from build123d import *
from build123d import SkipClean  # not in build123d's __all__

# Parameters (mm, degrees)
F0_R         = 8.117177454
F1_DEPTH     = 25
F2_SIZE      = 3
F3_DEPTH     = 25
F4_SIZE      = 5
F5_T4_DEPTH  = 109.868464735
F5_S5_R      = 25
F5_T6_DEPTH  = 57
F5_T8_ANGLE  = 167.4336377222
F5_T12_DEPTH = 109.868464735
F5_S13_R     = 25
F5_T14_DEPTH = 57


# Not quite as in the source:
# - a fillet or chamfer that OpenCascade refuses, or shapes differently, is made with other operations: its cross-section is extruded or revolved along the edge and cut away or added


with BuildPart() as f1:
    # F0 (on Front) → F1 (new body)
    with BuildSketch(Plane.XZ):
        with BuildLine():
            ThreePointArc((5.4392563458, -24.4011165811), (19.5061709293, -15.6367930113), (25, 0))
            ThreePointArc((25, 0), (19.5061709293, 15.6367930113), (5.4392563458, 24.4011165811))
            ThreePointArc((5.4392563458, 24.4011165811), (-25, 0), (5.4392563458, -24.4011165811))
        make_face()
        Circle(F0_R, mode=Mode.SUBTRACT)
        with BuildLine():
            ThreePointArc((5.4392563458, 24.4011165811), (19.5061709293, 15.6367930113), (25, 0))
            ThreePointArc((25, 0), (19.5061709293, -15.6367930113), (5.4392563458, -24.4011165811))
            Line((5.4392563458, -24.4011165811), (91.6416380189, -14.909896868))
            ThreePointArc((91.6416380189, -14.909896868), (75, 0), (91.6416380189, 14.909896868))
            Line((91.6416380189, 14.909896868), (5.4392563458, 24.4011165811))
        make_face()
        with BuildLine():
            ThreePointArc((105, 0), (101.1719418698, 10.0093813424), (91.6416380189, 14.909896868))
            ThreePointArc((91.6416380189, 14.909896868), (75, 0), (91.6416380189, -14.909896868))
            ThreePointArc((91.6416380189, -14.909896868), (101.1719418698, -10.0093813424), (105, 0))
        make_face()
        with Locations((90, 0)):
            Circle(F0_R, mode=Mode.SUBTRACT)
    extrude(amount=F1_DEPTH)

    # F2
    f2_edges = [f1.edges().sort_by_distance(p)[0] for p in [
        (-25, -25, 0),
        (48.540447, -25, -19.655507),
        (105, -25, 0),
        (48.540447, -25, 19.655507),
        (-8.117177, -25, 0),
        (81.882823, -25, 0),
    ]]
    chamfer(f2_edges, length=F2_SIZE)

    # F0 (on Front) → F3 (join)
    with BuildSketch(Plane.XZ):
        with BuildLine():
            ThreePointArc((5.4392563458, -24.4011165811), (19.5061709293, -15.6367930113), (25, 0))
            ThreePointArc((25, 0), (19.5061709293, 15.6367930113), (5.4392563458, 24.4011165811))
            ThreePointArc((5.4392563458, 24.4011165811), (-25, 0), (5.4392563458, -24.4011165811))
        make_face()
        Circle(F0_R, mode=Mode.SUBTRACT)
    with SkipClean():  # cleaning this boolean's faces spoils the solid; the shape is the same uncleaned
        extrude(amount=-F3_DEPTH)

    # F4
    f4_edges = [f1.edges().sort_by_distance(p)[0] for p in [
        (-5.439256, 25, 24.401117),
        (-8.117177, 25, 0),
    ]]
    chamfer(f4_edges, length=F4_SIZE)

    # F5: chamfer of 3 on 1 edges, made by hand


with BuildPart() as f5_tool2:
    # F5_s3 → F5_t4 (new body)
    with BuildSketch(Plane(origin=(88.922009846, 0, -9.7906614225), x_dir=(0, 1, 0), z_dir=(-0.9939931245, 0, 0.1094425346))):
        Polygon((0, -21.8498281134), (-3, -24.8498281134), (0, -24.8498281134), align=None)
    extrude(amount=F5_T4_DEPTH)

    # F5_s5 → F5_t6 (cut, symmetric)
    with BuildSketch(Plane.XZ.offset(1.5)):
        Circle(F5_S5_R)
    extrude(amount=F5_T6_DEPTH, both=True, mode=Mode.SUBTRACT)


with BuildPart() as f1_1:
    add(f1.part, clean=False)

    # F5_t1: cut F5_tool2
    add(f5_tool2.part, mode=Mode.SUBTRACT)

    # F5_s7 → F5_t8 (revolve, cut)
    with BuildSketch(Plane(origin=(88.922009846, 0, 9.7906614225), x_dir=(0, 1, 0), z_dir=(-0.9939931245, 0, -0.1094425346))):
        Polygon((0, 21.8498281134), (-3, 24.8498281134), (0, 24.8498281134), align=None)
    revolve(axis=Axis((90, 0, 0), (0, -1, 0)), revolution_arc=F5_T8_ANGLE, mode=Mode.SUBTRACT)


with BuildPart() as f5_tool10:
    # F5_s11 → F5_t12 (new body)
    with BuildSketch(Plane(origin=(-20.2864887038, 0, -2.2336218299), x_dir=(0, 1, 0), z_dir=(0.9939931245, 0, 0.1094425346))):
        Polygon((0, -21.8498281134), (-3, -24.8498281134), (0, -24.8498281134), align=None)
    extrude(amount=F5_T12_DEPTH)

    # F5_s13 → F5_t14 (cut, symmetric)
    with BuildSketch(Plane.XZ.offset(1.5)):
        Circle(F5_S13_R)
    extrude(amount=F5_T14_DEPTH, both=True, mode=Mode.SUBTRACT)


with BuildPart() as f1_2:
    add(f1_1.part, clean=False)

    # F5_t9: cut F5_tool10
    add(f5_tool10.part, mode=Mode.SUBTRACT)


solid = f1_2.part
CAD build for the part. Positions are in the model's coordinates, mm. Give positions to 0.01 mm unless a question says otherwise; leave off trailing zeros. Write each loop counter-clockwise with the first axis right and the second up, starting at its lowest first coordinate (ties: lowest second). Pieces come first, ordered by that corner, then holes. Notation, with made-up numbers: M 74.25,-13 L 116.25,-13 A27 ccw 116.25,23 Z; hole C 61,-14 d10. An arc over 180 degrees is marked long. Put each result on its own line as item: value. Start each with the question number.
(1) Band-saw the part on C-C, the plane x = 45.5. Write the cut outline in (y, z).
(2) Flat gauge pins, fed straight in: pin 1 Ø6 at (x, y) = (46, -3.5) entering from -Z; pin 2 Ø3 at (x, y) = (57.5, -16) entering from +Z; pin 3 Ø10 at (y, z) = (-15.5, -13.5) entering from -X. Where does each tip first touch, or does it go through?
(3) Band-saw the part on B-B, the plane y = -17.5. Write the cut outline in (x, z).
(4) Mould opens along Z. For faces 1 (the face through (81.89, -10.85, 0.36)), 2 (the face through (105, -12, 0)), 3 (the face through (49.14, -12.37, 19.59)), 4 (the face through (-1.8, -22.19, -8.11)) say: +Z half, -Z half, draft (parallel to the pull), parting line (faces both ways), or undercut.
(5) Band-saw the part on A-A, the plane x = 0. Write the cut outline in (y, z), and give its area (3 significant figures).
(6) Band-saw the part on D-D, the plane y = 18.5. Write the cut outline in (x, z).
(7) Probe L1, parallel to Z at x = 0, y = 14.75; L2, parallel to X at y = -21.5, z = -2; L3, parallel to Y at x = 37, z = -12.5. List the from-to ranges inside material, lowest first.
Response values:
1. outline: M -25,-16.97 L -22,-19.99 L -3,-19.99 L 0,-16.97 L 0,16.97 L -3,19.99 L -22,19.99 L -25,16.97 Z
2. pin 1: stops at z = -20.27
2. pin 2: stops at z = 18.83
2. pin 3: stops at x = -23.51
3. outline: M 5.44,-24.4 L 91.64,-14.91 A15 ccw 91.64,14.91 L 5.44,24.4 A25 ccw long Z; hole C 0,0 d16.23; hole C 90,0 d16.23
4. face 1: undercut
4. face 2: parting line
4. face 3: +Z half
4. face 4: undercut
5. outline: M -25,-22 L -22,-25 L 20,-25 L 25,-20 L 25,-13.12 L 20,-8.12 L -22,-8.12 L -25,-11.12 Z; M -25,11.12 L -22,8.12 L 20,8.12 L 25,13.12 L 25,20 L 20,25 L -22,25 L -25,22 Z
5. area: 1,620 mm2
6. outline: C 0,0 d50; hole C 0,0 d16.23
7. L1: z = -25 to -8.12, 8.12 to 25
7. L2: x = -24.92 to -7.87, 7.87 to 82.13, 97.87 to 104.87
7. L3: y = -25 to 0
